Part model, mm, in its own coordinate system. Round coordinates to 2 decimals unless told otherwise and drop trailing zeros. Loops run counter-clockwise (first coordinate to the right, second up) from the corner with the lowest first, then second, coordinate; pieces in that order, holes last.
(1) Cut at C-C on x = -1.75. List the corners of the cut face in (y, z) (3 decimals).
(2) Probe probe 1 along X at (y, z) = (-248.5, -4.5) (3 decimals); probe 2 along Y at (x, z) = (-2, -7) (3 decimals). List the from-to ranges inside material, lowest first.
(3) Cut at A-A on z = -1.5. List the corners of the cut face in (x, y) (3 decimals), then the cut area to 3 significant figures.
(4) Mould opens along Y. For faces 1 (the face through (-2, -958.85, 7)), 2 (the face through (0, -473, 9.525)), 3 (the face through (-2, 0, 7)) say: +Y half, -Y half, draft (parallel to the pull), parting line (faces both ways), or undercut.
(5) Flat gauge pins, fed straight in: pin 1 (1.6 mm diameter, centred on x = 8, y = -950, fed in from -Z); pin 2 (1 mm diameter, centred on x = -3, z = -4.5, fed in from -Y); pin 3 (1.6 mm diameter, centred on x = 0, z = -7.5, fed in from +Y) (3 decimals); pin 4 (4 mm diameter, centred on x = 6, z = -2, fed in from +Y). Where does each tip first touch, or does it go through?
(6) Cut at B-B on y = -295.5. List the corners of the cut face in (x, z) (3 decimals).
from build123d import *

# Parameters (mm, degrees)
F0_W     = 19.05
F0_H     = 19.05
F0_W_2   = 12.7
F0_H_2   = 12.7
F1_DEPTH = 958.85
F2_W     = 15.875
F2_H     = 3.175
F3_DEPTH = 19.05


with BuildPart() as f1:
    # F0 (on Front) → F1 (new body)
    with BuildSketch(Plane.XZ):
        Rectangle(F0_W, F0_H)
        Rectangle(F0_W_2, F0_H_2, mode=Mode.SUBTRACT)
    extrude(amount=F1_DEPTH)

    # F2 (on face) → F3 (cut)
    with BuildSketch(Plane(origin=(-9.525, 0, 0), x_dir=(0, -1, 0), z_dir=(-1, 0, 0))):
        with Locations((7.9375, -7.9375)):
            Rectangle(F2_W, F2_H)
        with Locations((950.9125, -7.9375)):
            Rectangle(F2_W, F2_H)
    extrude(amount=-F3_DEPTH, mode=Mode.SUBTRACT)


solid = f1.part
Final values:
1. outline: (-958.85, 6.35) - (0, 6.35) - (0, 9.525) - (-958.85, 9.525) - close; (-942.975, -9.525) - (-15.875, -9.525) - (-15.875, -6.35) - (-942.975, -6.35) - close
2. probe 1: x = -9.525 to -6.35, 6.35 to 9.525
2. probe 2: y = -942.975 to -15.875
3. outline: (-9.525, -958.85) - (-6.35, -958.85) - (-6.35, 0) - (-9.525, 0) - close; (6.35, -958.85) - (9.525, -958.85) - (9.525, 0) - (6.35, 0) - close
3. area: 6,090 mm2
4. face 1: -Y half
4. face 2: draft
4. face 3: +Y half
5. pin 1: stops at z = -6.35
5. pin 2: passes through
5. pin 3: stops at y = -15.875
5. pin 4: stops at y = 0
6. outline: (-9.525, -9.525) - (9.525, -9.525) - (9.525, 9.525) - (-9.525, 9.525) - close; hole (-6.35, -6.35) - (6.35, -6.35) - (6.35, 6.35) - (-6.35, 6.35) - close
